Here's the drawing with two shaded views (mm, measured from the low corner). I have some questions. A direction names the side the tool comes from. Coordinates: 2 decimals unless noted, no trailing zeros. Write each loop counter-clockwise with the first axis right and the second up, starting at its lowest first coordinate (ties: lowest second). Pieces come first, ordered by that corner, then holes. Notation, with made-up numbers: (11.5, -12.5) -> (47.5, -12.5) arc R21 cw to (47.5, 11.5) -> close; hole circle Ø6 at (3, 42.5). An arc over 180 degrees is marked (long way). Put each result on its own line as item: value.
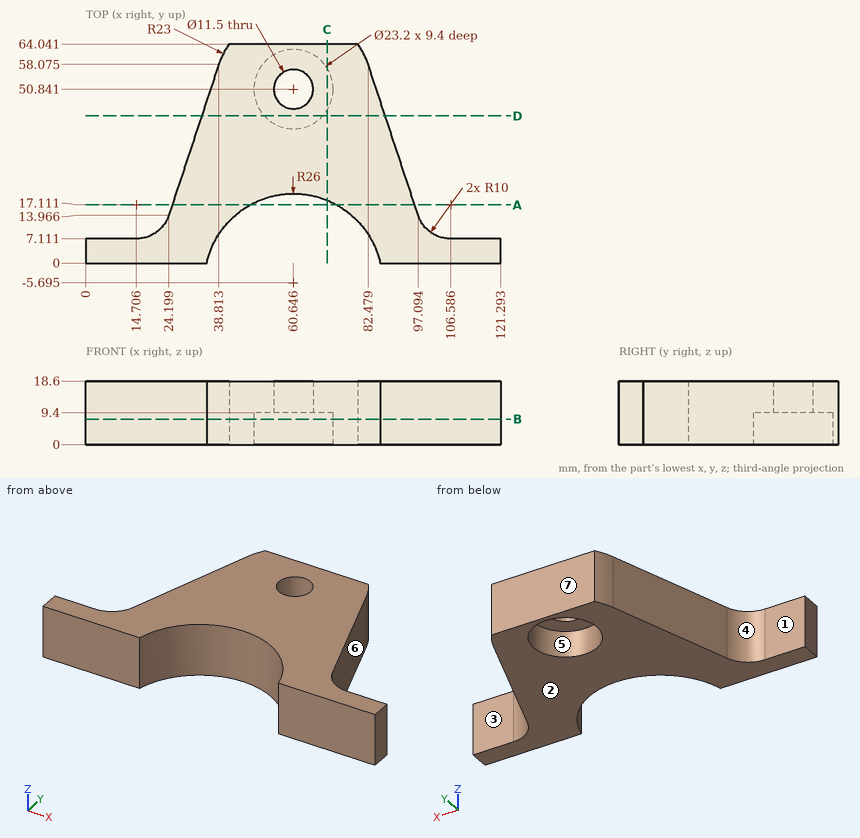
Item 1: Imagine slicing it at A-A on y = 17. Write out the boundary of the cut face in (x, z) (1 decimal).
Output:
outline: (25.2, 0) -> (48, 0) -> (48, 18.6) -> (25.2, 18.6) -> close; (73.3, 0) -> (96.1, 0) -> (96.1, 18.6) -> (73.3, 18.6) -> close
Item 2: For P1, Ø5, axis at y = 56, z = 16, coming from the -X side; P2, Ø6, axis at x = 40, z = 11, coming from the -Y side (1 decimal); P3, Ø7, axis at x = 66, y = 52.5, coming from the -Z side; P4, Ø9, axis at x = 60.65, y = 50.84, coming from the +Z side, each with a flat end and sliding along its axis, tell me the tip position at first contact or that it passes through.
Output:
P1: stops at x = 37.3
P2: stops at y = 5.1
P3: stops at z = 9.4
P4: passes through
Item 3: Please list where these lines run through material, in increasing order: line 1 along X through (y, z) = (11, 9.75) (1 decimal); line 2 along Y through (x, z) = (110.5, 4.5); line 3 along X through (y, z) = (55, 16) (1 decimal). Write a range as from..to.
Output:
line 1: x = 22.6..40.7, 80.6..98.7
line 2: y = 0..7.11
line 3: x = 37.8..56.7, 64.6..83.5
Item 4: Which directions (+Z, -Z, +X, -X, +Y, -Y) give clear straight access to the entire face, cutting with the end or side of a thin tool? Please do the marked faces 1, 2 and 3.
Output:
face 1: +Z, -Z, -X, +Y
face 2: -Z, +X, -X, +Y, -Y
face 3: +Z, -Z, +X, +Y
Item 5: If we mould it in two halves opening along X, with no side actions, what happens to the marked faces 4, 5, 6 and 7? For each: released by +X, released by -X, zero draft, split by the parting line, or undercut.
Output:
face 4: released by -X
face 5: undercut
face 6: released by +X
face 7: zero draft
Item 6: Imagine slicing it at B-B on z = 7.5. Write out the boundary of the cut face in (x, y) (1 decimal).
Output:
outline: (0, 0) -> (35.3, 0) arc R26 cw to (86, 0) -> (121.3, 0) -> (121.3, 7.1) -> (106.6, 7.1) arc R10 cw to (97.1, 14) -> (82.5, 58.1) arc R23 ccw to (79.5, 64) -> (41.8, 64) arc R23 ccw to (38.8, 58.1) -> (24.2, 14) arc R10 cw to (14.7, 7.1) -> (0, 7.1) -> close; hole circle Ø23.2 at (60.6, 50.8)
Item 7: Imagine slicing it at D-D on y = 43. Write out the boundary of the cut face in (x, z) (1 decimal).
Output:
outline: (33.8, 0) -> (52.1, 0) -> (52.1, 9.4) -> (69.2, 9.4) -> (69.2, 0) -> (87.5, 0) -> (87.5, 18.6) -> (33.8, 18.6) -> close
Item 8: Imagine slicing it at C-C on x = 70.5. Write out the boundary of the cut face in (y, z) (1 decimal).
Output:
outline: (18.4, 0) -> (44.7, 0) -> (44.7, 9.4) -> (57, 9.4) -> (57, 0) -> (64, 0) -> (64, 18.6) -> (18.4, 18.6) -> close
